from build123d import *

# Parameters (mm, degrees)
SKETCH1_W           = 55
SKETCH1_H           = 95
BOSS_EXTRUDE1_DEPTH = 30
SKETCH2_W           = 52.6
SKETCH2_H           = 92.6
CUT_EXTRUDE1_DEPTH  = 28.8
SKETCH3_R           = 3.5
BOSS_EXTRUDE2_DEPTH = 16
SKETCH6_R           = 1.6
BOSS_EXTRUDE3_DEPTH = 1.5
FILLET3_R           = 2
SKETCH8_W           = 44.2
SKETCH8_H           = 32.4
BOSS_EXTRUDE4_DEPTH = 10
SKETCH9_W           = 43
SKETCH9_H           = 30
CUT_EXTRUDE3_DEPTH  = 10
CUT_EXTRUDE4_REACH  = 97
SKETCH11_W          = 8
SKETCH11_H          = 3
SKETCH7_R           = 1.2
CUT_EXTRUDE5_DEPTH  = 16


with BuildPart() as part:
    # Sketch1 → Boss-Extrude1 (new body)
    with BuildSketch(Plane.XY):
        with Locations((27.5, -47.5)):
            Rectangle(SKETCH1_W, SKETCH1_H)
    extrude(amount=BOSS_EXTRUDE1_DEPTH)

    # Sketch2 → Cut-Extrude1 (cut)
    with BuildSketch(Plane(origin=(0, 0, 0), x_dir=(-1, 0, 0), z_dir=(0, 0, -1))):
        with Locations((-27.5, -47.5)):
            Rectangle(SKETCH2_W, SKETCH2_H)
    extrude(amount=-CUT_EXTRUDE1_DEPTH, mode=Mode.SUBTRACT)

    # Sketch3 → Boss-Extrude2 (add)
    with BuildSketch(Plane(origin=(0, 0, 28.8), x_dir=(-1, 0, 0), z_dir=(0, 0, -1))):
        with Locations((-4.2, -4.2)):
            Circle(SKETCH3_R)
        with Locations((-48.2, -4.2)):
            Circle(SKETCH3_R)
        with Locations((-48.2, -88.2)):
            Circle(SKETCH3_R)
        with Locations((-4.2, -88.2)):
            Circle(SKETCH3_R)
    extrude(amount=BOSS_EXTRUDE2_DEPTH)

    # Sketch6 → Boss-Extrude3 (add)
    with BuildSketch(Plane(origin=(0, 0, 12.8), x_dir=(-1, 0, 0), z_dir=(0, 0, -1))):
        with Locations((-4.2, -4.2)):
            Circle(SKETCH6_R)
        with Locations((-48.2, -4.2)):
            Circle(SKETCH6_R)
        with Locations((-48.2, -88.2)):
            Circle(SKETCH6_R)
        with Locations((-4.2, -88.2)):
            Circle(SKETCH6_R)
    extrude(amount=BOSS_EXTRUDE3_DEPTH)

    # Fillet3
    fillet3_edges = [part.edges().sort_by_distance(p)[0] for p in [
        (0, 0, 15),
        (55, 0, 15),
        (55, -95, 15),
        (0, -95, 15),
    ]]
    fillet(fillet3_edges, radius=FILLET3_R)

    # Sketch8 → Boss-Extrude4 (add)
    with BuildSketch(Plane(origin=(0, 0, 28.8), x_dir=(-1, 0, 0), z_dir=(0, 0, -1))):
        with Locations((-31.7, -37.4)):
            Rectangle(SKETCH8_W, SKETCH8_H)
    extrude(amount=BOSS_EXTRUDE4_DEPTH)

    # Sketch9 → Cut-Extrude3 (cut)
    with BuildSketch(Plane(origin=(0, 0, 18.8), x_dir=(-1, 0, 0), z_dir=(0, 0, -1))):
        with Locations((-32.3, -37.4)):
            Rectangle(SKETCH9_W, SKETCH9_H)
    extrude(amount=-CUT_EXTRUDE3_DEPTH, mode=Mode.SUBTRACT)

    # Sketch11 → Cut-Extrude4 (cut, up to next)
    with BuildSketch(Plane(origin=(0, 0, 0), x_dir=(1, 0, 0), z_dir=(0, 1, 0)), mode=Mode.PRIVATE) as cut_extrude4_sk1:
        with Locations((41.2, -9.68)):
            Rectangle(SKETCH11_W, SKETCH11_H)
    cut_extrude4_tool1 = extrude(cut_extrude4_sk1.sketch, amount=-CUT_EXTRUDE4_REACH, mode=Mode.PRIVATE) & part.part
    add(cut_extrude4_tool1.solids().sort_by_distance((41.2, 0, 9.68))[0], mode=Mode.SUBTRACT)

    # Sketch7 → Cut-Extrude5 (cut)
    with BuildSketch(Plane(origin=(0, 0, 11.3), x_dir=(-1, 0, 0), z_dir=(0, 0, -1))):
        with Locations((-4.2, -4.2)):
            Circle(SKETCH7_R)
        with Locations((-48.2, -4.2)):
            Circle(SKETCH7_R)
        with Locations((-48.2, -88.2)):
            Circle(SKETCH7_R)
        with Locations((-4.2, -88.2)):
            Circle(SKETCH7_R)
    extrude(amount=-CUT_EXTRUDE5_DEPTH, mode=Mode.SUBTRACT)


solid = part.part
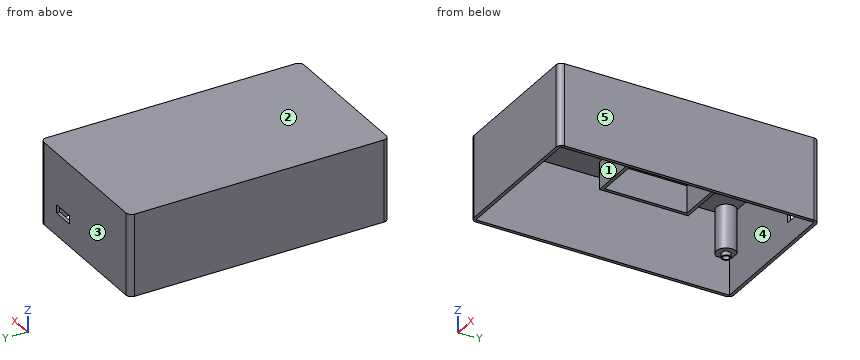
Could you check a few things on this model? Use its own coordinates, in mm. Face numbers are marked on the shaded views. A direction names the side the tool comes from. Give positions to 0.01 mm unless a question says otherwise; leave off trailing zeros. Order: outer loops, then holes, each group sorted by start corner. A loop starts at its lowest first (then second) coordinate and runs counter-clockwise, first axis right, second up.
1. Which directions (+Z, -Z, +X, -X, +Y, -Y) give clear straight access to the entire face, cutting with the end or side of a thin tool? Please do the marked faces 1 and 2.
Answers below:
face 1: -Z
face 2: +Z, +X, -X, +Y, -Y
2. I need wall thicknesses on L1, parallel to Y at x = 19.5, z = 28.5; L2, parallel to X at y = -41, z = 25; L3, parallel to Y at x = 4.2, z = 20.25. Which ranges of each line are inside material? Lowest first, please.
Answers below:
L1: y = -95 to -93.8, -53.6 to -52.4, -22.4 to -21.2, -1.2 to 0
L2: x = 0 to 1.2, 9.6 to 10.8, 53.8 to 55
L3: y = -95 to -93.8, -91.7 to -89.4, -87 to -84.7, -7.7 to -5.4, -3 to 0
3. For pin 1 (1.3 mm diameter, centred on x = 2, y = -2, fed in from -Z); pin 2 (5 mm diameter, centred on x = 39.5, y = -15, fed in from -Z); pin 3 (1.9 mm diameter, centred on x = 48.5, y = -4.5, fed in from -Z), each with a flat end and sliding along its axis, tell me the tip position at first contact or that it passes through.
Answers below:
pin 1: stops at z = 12.8
pin 2: stops at z = 28.8
pin 3: stops at z = 11.3
4. Suppose I cut it at C-C (z = 22). State how many separate pieces and enclosed holes the cut face has, plus the area to 3 significant figures.
Answers below:
separate pieces: 2
enclosed holes: 7
area: 624 mm2
5. Suppose I cut it at A-A (z = 5). Write out the boundary of the cut face in (x, y).
Answers below:
outline: (0, -93) arc R2 ccw to (2, -95) - (53, -95) arc R2 ccw to (55, -93) - (55, -2) arc R2 ccw to (53, 0) - (2, 0) arc R2 ccw to (0, -2) - close; hole (1.2, -93.8) - (53.8, -93.8) - (53.8, -1.2) - (1.2, -1.2) - close
6. Suppose I cut it at D-D (x = 28.5). Write out the boundary of the cut face in (y, z), plus the area to 3 significant figures.
Answers below:
outline: (-95, 0) - (-93.8, 0) - (-93.8, 28.8) - (-53.6, 28.8) - (-53.6, 18.8) - (-52.4, 18.8) - (-52.4, 28.8) - (-22.4, 28.8) - (-22.4, 18.8) - (-21.2, 18.8) - (-21.2, 28.8) - (-1.2, 28.8) - (-1.2, 0) - (0, 0) - (0, 30) - (-95, 30) - close
area: 207 mm2
7. Thinking about a two-plate mould opening in Y: for the marked faces 3, 4 and 5, which applies, +Y half, -Y half, draft (parallel to the pull), parting line (faces both ways), or undercut?
Answers below:
face 3: +Y half
face 4: undercut
face 5: draft
